Input: part model. Units: mm. Frame: model coordinates. A direction names the side the tool comes from. Round coordinates to 2 decimals unless told otherwise and drop trailing zeros. Loops run counter-clockwise (first coordinate to the right, second up) from the corner with the lowest first, then second, coordinate; pieces in that order, holes last. Notation, with made-up numbers: (54, -6) - (97, -6) arc R24 cw to (97, 31) - close; hole circle Ø10 at (88, 85.25). An arc over 180 degrees is marked (long way). Use CSV: the item, a comma, the result in double quotes. Start each with the question number.
1. Access query for faces 1 (the flat face through (-10, 4, 4)), 2 (the flat face through (2.834, 13, -2)), 3 (the flat face through (7, 25, 2)), 4 (the flat face through (5, 16.583, -2)), 5 (the flat face through (-5, -23.678, -2)). Directions: +Z, -Z, +X, -X, +Y, -Y. A direction counts if a zero-diameter tool reaches every point of the face in a straight line with its end or side. Return the directions, or none.
2. Material intervals for probe 1 along Y at (x, z) = (6.25, -1.25); probe 2 along Y at (x, z) = (9, 2.5); probe 3 along Y at (x, z) = (-9.75, 2.25), sorted ascending. Write a range as from..to.
3. Cut plane D-D (x = -6.5). Return loops of the section in (y, z).
4. Pin query (flat end, axial travel): P1, Ø3, axis at x = -6, z = -2, coming from the -Y side; P2, Ø1.6, axis at x = -0.5, z = 4, coming from the +Y side; P3, Ø3, axis at y = -20, z = -2, coming from the -X side; P4, Ø1.5, axis at y = 22.5, z = -1.5, coming from the +X side. Return the tip coordinate at first contact, or that it passes through.
5. Cut plane A-A (x = 2.25). Return loops of the section in (y, z), and give its area (3 significant figures).
6. Cut plane C-C (y = -20.5). Return loops of the section in (x, z), and give its area (3 significant figures).
7. Pull-direction query (Y, two-part tool) for faces 6 (the flat face through (7.852, 13, -2)), 7 (the flat face through (0, 5, 7)), 8 (the flat face through (-4, 25, 1)); classes: +Y half, -Y half, draft (parallel to the pull), parting line (faces both ways), or undercut.
8. Cut plane B-B (z = 2.5). Return loops of the section in (x, y).
```python
from build123d import *

# Parameters (mm, degrees)
F0_W          = 20
F0_H          = 27.3
F0_W_2        = 23
F0_H_2        = 14
F0_W_3        = 6.929286
F0_H_3        = 2.628351
F0_W_4        = 5.49564
F0_H_4        = 4.181466
F1_DEPTH      = 1.3
F0_W_5        = 4.898288
F0_H_5        = 5.973523
F0_W_6        = 5.017759
F0_H_6        = 7.765578
F2_DEPTH      = 7
F3_DEPTH      = 6.75
F0_W_7        = 6.6
F0_H_7        = 1.66
F4_DEPTH      = 3.5
F4_DEPTH_BACK = 3
F5_DEPTH      = 3.5
F6_R          = 3
F7_DEPTH      = 8


with BuildPart() as f1:
    # F0 (on Top) → F1 (new body)
    with BuildSketch(Plane.XY):
        Polygon((3.3, 25), (-11.5, 25), (-11.5, -11), (11.5, -11), (11.5, 25), (9.9, 25), align=None)
        with Locations((0, 4.65)):
            Rectangle(F0_W, F0_H, mode=Mode.SUBTRACT)
        with Locations((0, -18)):
            Rectangle(F0_W_2, F0_H_2)
        with Locations((-5.170625, -22.364168)):
            Rectangle(F0_W_3, F0_H_3, mode=Mode.SUBTRACT)
        with Locations((6.418009, -20.990259)):
            Rectangle(F0_W_4, F0_H_4, mode=Mode.SUBTRACT)
    extrude(amount=F1_DEPTH)

    # F0 (on Top) → F2 (join)
    with BuildSketch(Plane.XY):
        with Locations((0, 4.65)):
            Rectangle(F0_W, F0_H)
        with Locations((-5.827712, 3.919329)):
            Rectangle(F0_W_5, F0_H_5, mode=Mode.SUBTRACT)
        with Locations((5.342776, 12.700408)):
            Rectangle(F0_W_6, F0_H_6, mode=Mode.SUBTRACT)
        with Locations((-5.827712, 3.919329)):
            Rectangle(F0_W_5, F0_H_5)
        with Locations((5.342776, 12.700408)):
            Rectangle(F0_W_6, F0_H_6)
    extrude(amount=F2_DEPTH)

    # F0 (on Top) → F3 (join)
    with BuildSketch(Plane.XY):
        with Locations((0, -18)):
            Rectangle(F0_W_2, F0_H_2)
        with Locations((-5.170625, -22.364168)):
            Rectangle(F0_W_3, F0_H_3, mode=Mode.SUBTRACT)
        with Locations((6.418009, -20.990259)):
            Rectangle(F0_W_4, F0_H_4, mode=Mode.SUBTRACT)
        with Locations((6.418009, -20.990259)):
            Rectangle(F0_W_4, F0_H_4)
        with Locations((-5.170625, -22.364168)):
            Rectangle(F0_W_3, F0_H_3)
    extrude(amount=F3_DEPTH)

    # F0 (on Top) → F4 (join, two sides)
    with BuildSketch(Plane.XY) as f4_sk:
        with Locations((6.6, 25.83)):
            Rectangle(F0_W_7, F0_H_7)
    extrude(amount=F4_DEPTH)
    extrude(f4_sk.sketch, amount=-F4_DEPTH_BACK)

    # F0 (on Top) → F5 (join)
    with BuildSketch(Plane.XY):
        with Locations((5.342776, 12.700408)):
            Rectangle(F0_W_6, F0_H_6)
        with Locations((-5.827712, 3.919329)):
            Rectangle(F0_W_5, F0_H_5)
        with Locations((6.418009, -20.990259)):
            Rectangle(F0_W_4, F0_H_4)
        with Locations((-5.170625, -22.364168)):
            Rectangle(F0_W_3, F0_H_3)
    extrude(amount=-F5_DEPTH)

    # F6 (on face) → F7 (join)
    with BuildSketch(Plane(origin=(0, 26.66, 0), x_dir=(-1, 0, 0), z_dir=(0, 1, 0))):
        with Locations((-6.6, 0.25)):
            Circle(F6_R)
    extrude(amount=F7_DEPTH)


solid = f1.part
```
Established:
1,face 1,"+Z, -X, +Y"
1,face 2,"-Z, -X, +Y, -Y"
1,face 3,"+Z, +X, -X"
1,face 4,"-Z, +X, -X"
1,face 5,"-Z, +X, -X, -Y"
2,probe 1,"y = -23.08..-18.9, 8.82..16.58, 25..34.66"
2,probe 2,"y = -25..-11, -9..18.3, 25..26.66"
2,probe 3,"y = -25..-11, -9..18.3"
3,outline,"(-25, 0) - (-23.68, 0) - (-23.68, -3.5) - (-21.05, -3.5) - (-21.05, 0) - (0.93, 0) - (0.93, -3.5) - (6.91, -3.5) - (6.91, 0) - (25, 0) - (25, 1.3) - (18.3, 1.3) - (18.3, 7) - (-9, 7) - (-9, 1.3) - (-11, 1.3) - (-11, 6.75) - (-25, 6.75) - close"
4,P1,"stops at y = -23.68"
4,P2,"stops at y = 18.3"
4,P3,"stops at x = -8.64"
4,P4,"passes through"
5,outline,"(-25, 0) - (25, 0) - (25, 1.3) - (18.3, 1.3) - (18.3, 7) - (-9, 7) - (-9, 1.3) - (-11, 1.3) - (-11, 6.75) - (-25, 6.75) - close"
5,area,"297 mm2"
6,outline,"(-11.5, 0) - (3.67, 0) - (3.67, -3.5) - (9.17, -3.5) - (9.17, 0) - (11.5, 0) - (11.5, 6.75) - (-11.5, 6.75) - close"
6,area,"174 mm2"
7,face 6,"undercut"
7,face 7,"draft"
7,face 8,"+Y half"
8,outline,"(-11.5, -25) - (11.5, -25) - (11.5, -11) - (-11.5, -11) - close; (-10, -9) - (10, -9) - (10, 18.3) - (-10, 18.3) - close; (3.3, 25) - (9.9, 25) - (9.9, 26.66) - (8.58, 26.66) - (8.58, 34.66) - (4.62, 34.66) - (4.62, 26.66) - (3.3, 26.66) - close"
